The model under review builds one solid part; all positions refer to its coordinate system, in mm. Face numbers are marked on the shaded views. Coordinates: 2 decimals unless noted, no trailing zeros. Write each loop counter-clockwise with the first axis right and the second up, starting at its lowest first coordinate (ties: lowest second). Pieces come first, ordered by that corner, then holes. Notation, with made-up numbers: (-27, -23.75) - (-14, -23.75) arc R14 cw to (-14, -19.75) - close; hole circle Ø5 at (3.25, 35). An arc over 180 degrees is marked (long way). Return JSON: item names as keys, results as strings. Group by question number.
(1) For pin 1 Ø6 at (y, z) = (-19.5, -46) entering from +X; pin 2 Ø2 at (y, z) = (-88, 20.5) entering from +X; pin 3 Ø6 at (y, z) = (-12.5, 19) entering from +X, all flat-tipped, find the tip position at first contact; note any pin that passes through.
(2) To check wall thickness, follow L1, parallel to Z at x = 0, y = -2; L2, parallel to Y at x = 84, z = -21.5; L3, parallel to Z at x = 28, y = -50.5. State the ranges of each line that lie inside material, in increasing order. Write a range as from..to.
(3) Draft analysis for pull direction Z (two halves, no side actions). For the marked faces 1, 2 and 3, state which applies: released by +Z, released by -Z, zero draft, split by the parting line, or undercut.
(4) We need section C-C on x = -22.5. State the section outline as (y, z) points.
(5) We need section D-D on y = -20. State the section outline as (x, z) points, then the cut area to 3 significant figures.
(6) We need section A-A on z = 0. State the section outline as (x, y) points.
(7) We need section B-B on x = 0. State the section outline as (y, z) points.
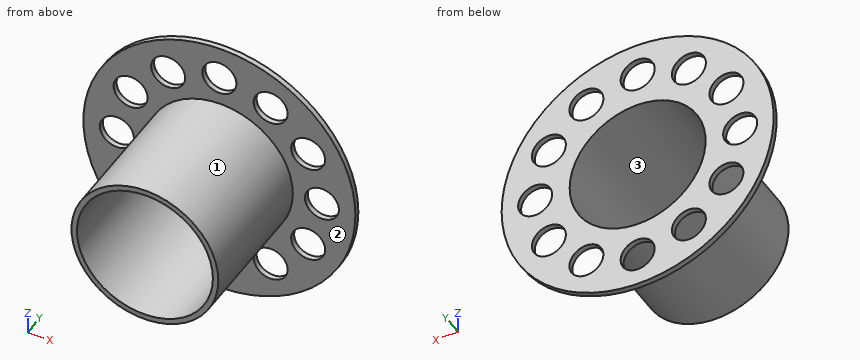
```python
from build123d import *

# Parameters (mm, degrees)
F0_R     = 100
F0_R_2   = 12.5
F0_R_3   = 50
F1_DEPTH = 4
F2_R     = 54
F2_R_2   = 50
F3_DEPTH = 100


with BuildPart() as f1:
    # F0 (on Front) → F1 (new body)
    with BuildSketch(Plane.XZ):
        Circle(F0_R)
        with Locations((-37.684567, -65.271585)):
            Circle(F0_R_2, mode=Mode.SUBTRACT)
        with Locations((-65.271585, -37.684567)):
            Circle(F0_R_2, mode=Mode.SUBTRACT)
        with Locations((0, -75.369135)):
            Circle(F0_R_2, mode=Mode.SUBTRACT)
        with Locations((37.684567, -65.271585)):
            Circle(F0_R_2, mode=Mode.SUBTRACT)
        with Locations((65.271585, -37.684567)):
            Circle(F0_R_2, mode=Mode.SUBTRACT)
        with Locations((-75.369135, 0)):
            Circle(F0_R_2, mode=Mode.SUBTRACT)
        with Locations((-65.271585, 37.684567)):
            Circle(F0_R_2, mode=Mode.SUBTRACT)
        with Locations((-37.684567, 65.271585)):
            Circle(F0_R_2, mode=Mode.SUBTRACT)
        Circle(F0_R_3, mode=Mode.SUBTRACT)
        with Locations((75.369135, 0)):
            Circle(F0_R_2, mode=Mode.SUBTRACT)
        with Locations((65.271585, 37.684567)):
            Circle(F0_R_2, mode=Mode.SUBTRACT)
        with Locations((37.684567, 65.271585)):
            Circle(F0_R_2, mode=Mode.SUBTRACT)
        with Locations((0, 75.369135)):
            Circle(F0_R_2, mode=Mode.SUBTRACT)
    extrude(amount=F1_DEPTH)

    # F2 (on face) → F3 (join)
    with BuildSketch(Plane.XZ.offset(4)):
        Circle(F2_R)
        Circle(F2_R_2, mode=Mode.SUBTRACT)
    extrude(amount=F3_DEPTH)


solid = f1.part
```
Ans:
{
 "1": {"pin 1": "x = 32.66", "pin 2": "x = 50.36", "pin 3": "x = 51.58"},
 "2": {"L1": "-100..-87.87, -62.87..-50, 50..62.87, 87.87..100", "L2": "-4..0", "L3": "-46.17..-41.42, 41.42..46.17"},
 "3": {"face 1": "split by the parting line", "face 2": "zero draft", "face 3": "undercut"},
 "4": {"outline": "(-104, -49.09) - (-4, -49.09) - (-4, -97.44) - (0, -97.44) - (0, -44.65) - (-104, -44.65) - close; (-104, 44.65) - (0, 44.65) - (0, 97.44) - (-4, 97.44) - (-4, 49.09) - (-104, 49.09) - close"},
 "5": {"outline": "circle Ø108 at (0, 0); hole circle Ø100 at (0, 0)", "area": "1,310 mm²"},
 "6": {"outline": "(-100, -4) - (-87.87, -4) - (-87.87, 0) - (-100, 0) - close; (-62.87, -4) - (-54, -4) - (-54, -104) - (-50, -104) - (-50, 0) - (-62.87, 0) - close; (50, -104) - (54, -104) - (54, -4) - (62.87, -4) - (62.87, 0) - (50, 0) - close; (87.87, -4) - (100, -4) - (100, 0) - (87.87, 0) - close"},
 "7": {"outline": "(-104, -54) - (-4, -54) - (-4, -62.87) - (0, -62.87) - (0, -50) - (-104, -50) - close; (-104, 50) - (0, 50) - (0, 62.87) - (-4, 62.87) - (-4, 54) - (-104, 54) - close; (-4, -100) - (0, -100) - (0, -87.87) - (-4, -87.87) - close; (-4, 87.87) - (0, 87.87) - (0, 100) - (-4, 100) - close"}
}
